Verification items for this drawing (mm, ordinates from the low corner). Round coordinates to 2 decimals unless told otherwise and drop trailing zeros. Order: outer loops, then holes, each group sorted by start corner. A loop starts at its lowest first (then second) coordinate and runs counter-clockwise, first axis right, second up. Notation, with made-up numbers: M 31.5,-21 L 85.5,-21 A28 ccw 85.5,4 Z; hole C 35,49 d1. An arc over 180 degrees is marked long. One line per item, written item: value. Start each with the question number.
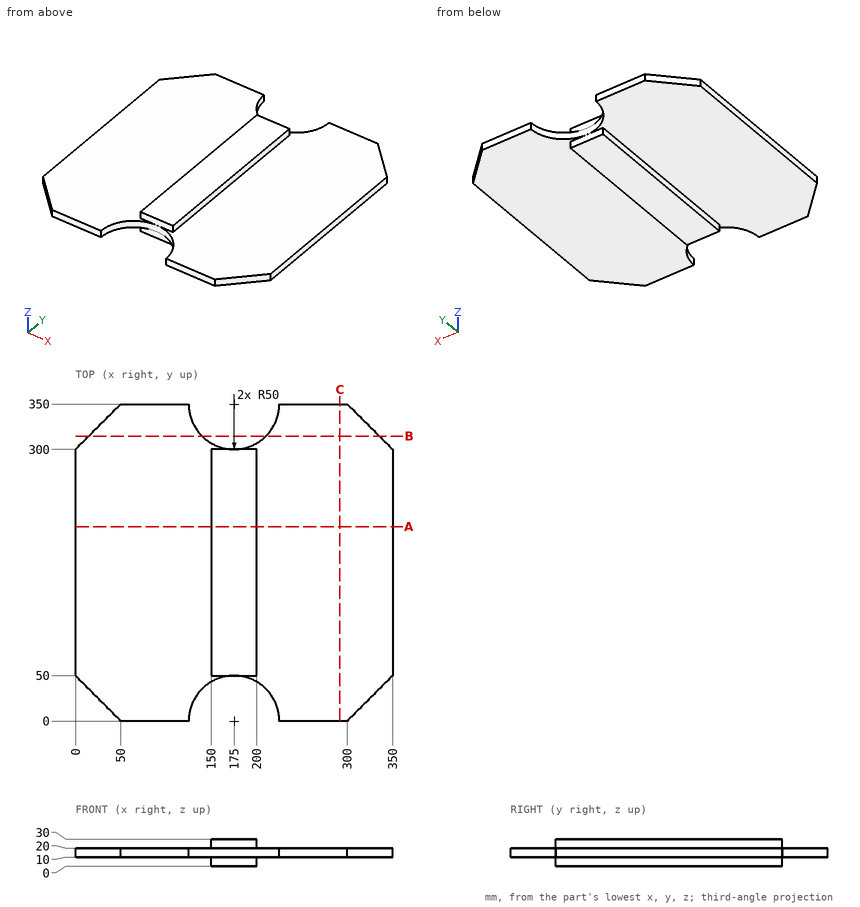
1. Section check A-A (y = 214.5). Record the cut outline in (x, z).
2. Section check B-B (y = 314.5). Record the cut outline in (x, z).
3. Scan lines: line 1 along X through (y, z) = (205, 28.75); line 2 along Y through (x, z) = (190, 5); line 3 along X through (y, z) = (29, 18.5). Record each from-to range of solid material in increasing order.
4. Depth check by flat-ended pin: pin 1 (3 mm diameter, centred on y = 211, z = 6.5, fed in from +X); pin 2 (3 mm diameter, centred on y = 97.5, z = 22, fed in from -X); pin 3 (8 mm diameter, centred on x = 299.5, y = 211.5, fed in from -Z). Enter the tip coordinate at first touch or a pass-through.
5. Section check C-C (x = 292). Record the cut outline in (y, z).
Geometry check:
1. outline: M 0,10 L 150,10 L 150,0 L 200,0 L 200,10 L 350,10 L 350,20 L 200,20 L 200,30 L 150,30 L 150,20 L 0,20 Z
2. outline: M 14.5,10 L 139.79,10 L 139.79,20 L 14.5,20 Z; M 210.21,10 L 335.5,10 L 335.5,20 L 210.21,20 Z
3. line 1: x = 150 to 200
3. line 2: y = 50 to 300
3. line 3: x = 21 to 134.27, 215.73 to 329
4. pin 1: stops at x = 200
4. pin 2: stops at x = 150
4. pin 3: stops at z = 10
5. outline: M 0,10 L 350,10 L 350,20 L 0,20 Z
